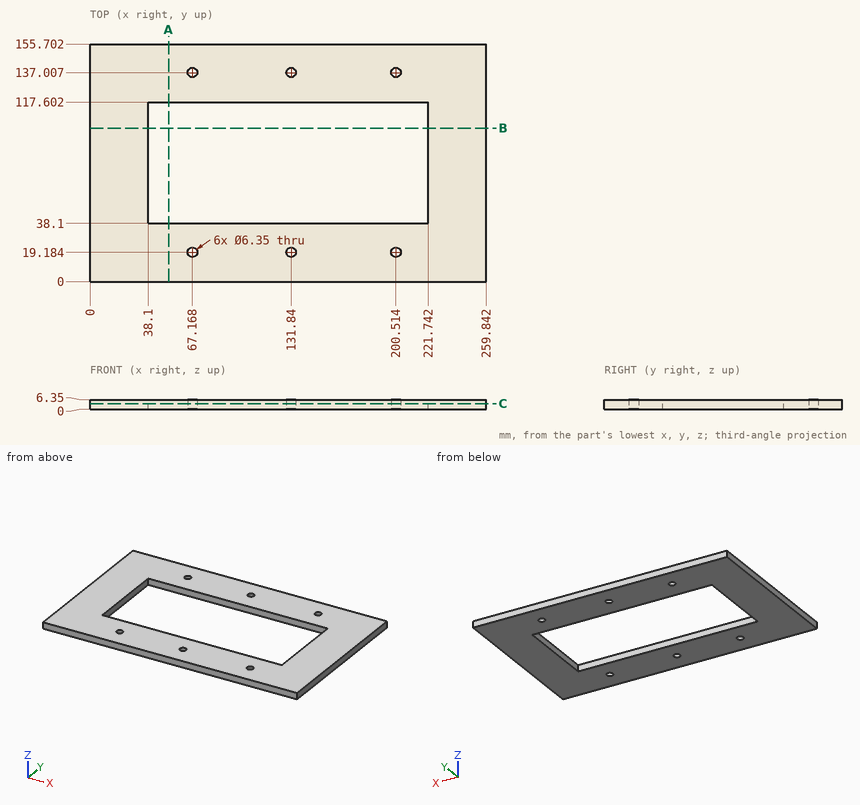
Design review of the part shown in the three views and the two pictorial views. Dimensions are in mm from the part's minimum x, y and z. Round coordinates to 2 decimals unless told otherwise and drop trailing zeros. Order: outer loops, then holes, each group sorted by start corner. A loop starts at its lowest first (then second) coordinate and runs counter-clockwise, first axis right, second up. Notation, with made-up numbers: (71, 73) -> (121, 73) arc R27 cw to (121, 99) -> close; hole circle Ø5 at (55, -5.5). An arc over 180 degrees is marked (long way). Write item = value, one per line. Start each with the question number.
1) Take a section at B-B on y = 100.5. State the section outline as (x, z) points.
2) Take a section at A-A on x = 51.5. State the section outline as (y, z) points.
3) To check wall thickness, follow line 1 (X direction, y = 38.5, z = 0.75); line 2 (Y direction, x = 154, z = 1.25); line 3 (Y direction, x = 198, z = 3.5) (1 decimal). State the ranges of each line that lie inside material, in increasing order. Write a range as from..to.
4) Take a section at C-C on z = 3.75. Count the separate pieces of the cut face and the enclosed holes in it, plus the area to 3 significant figures.
Verdict:
q1.outline = (0, 0) -> (38.1, 0) -> (38.1, 6.35) -> (0, 6.35) -> close; (221.74, 0) -> (259.84, 0) -> (259.84, 6.35) -> (221.74, 6.35) -> close
q2.outline = (0, 0) -> (38.1, 0) -> (38.1, 6.35) -> (0, 6.35) -> close; (117.6, 0) -> (155.7, 0) -> (155.7, 6.35) -> (117.6, 6.35) -> close
q3.line_1 = 0..38.1, 221.74..259.84
q3.line_2 = 0..38.1, 117.6..155.7
q3.line_3 = 0..17.2, 21.1..38.1, 117.6..135.1, 138.9..155.7
q4.separate_pieces = 1
q4.enclosed_holes = 7
q4.area = 25,700 mm2
